from build123d import *

# Parameters (mm, degrees)
EXTRUDE_1_DEPTH          = 4
CUT_EXTRUDE_1_DEPTH      = 3
SKETCH_4_R               = 2.6
CUT_EXTRUDE_9_DEPTH      = 19
CUT_EXTRUDE_9_DEPTH_BACK = 2
SKETCH_5_W               = 0.2
SKETCH_5_H               = 8
CUT_EXTRUDE_11_DEPTH     = 5


with BuildPart() as part:
    # 草圖1 → 填料-伸長1 (new body)
    with BuildSketch(Plane.XY):
        with BuildLine():
            Line((-9, 0), (-9, 43))
            ThreePointArc((-9, 43), (0, 52), (9, 43))
            Line((9, 43), (9, 0))
            Line((9, 0), (-9, 0))
        make_face()
    extrude(amount=EXTRUDE_1_DEPTH)

    # 草圖2 → 除料-伸長1 (cut)
    with BuildSketch(Plane.XY.offset(4)):
        with BuildLine():
            Line((-2.6, 47.145110573), (-5, 33.352358854))
            ThreePointArc((-5, 33.352358854), (-6.5, 29.199046922), (-5, 25.045734991))
            Line((-5, 25.045734991), (-2.656326538, 11.243300615))
            ThreePointArc((-2.656326538, 11.243300615), (0, 9), (2.656326538, 11.243300615))
            Line((2.656326538, 11.243300615), (5, 25.045734991))
            ThreePointArc((5, 25.045734991), (6.5, 29.199046922), (5, 33.352358854))
            Line((5, 33.352358854), (2.6, 47.145110573))
            ThreePointArc((2.6, 47.145110573), (0, 49.331766334), (-2.6, 47.145110573))
        make_face()
    extrude(amount=-CUT_EXTRUDE_1_DEPTH, mode=Mode.SUBTRACT)

    # 草圖4 → 除料-伸長9 (cut, two sides)
    with BuildSketch(Plane.XY) as cut_extrude_9_sk:
        with Locations((0, 29.065156497)):
            Circle(SKETCH_4_R)
    extrude(amount=CUT_EXTRUDE_9_DEPTH, mode=Mode.SUBTRACT)
    extrude(cut_extrude_9_sk.sketch, amount=-CUT_EXTRUDE_9_DEPTH_BACK, mode=Mode.SUBTRACT)

    # 草圖5 → 除料-伸長11 (cut, through all)
    with BuildSketch(Plane.XY):
        with Locations((0, 4)):
            Rectangle(SKETCH_5_W, SKETCH_5_H)
    extrude(amount=CUT_EXTRUDE_11_DEPTH, mode=Mode.SUBTRACT)


solid = part.part
Work out the finished part from the listing and answer in its coordinate system (mm). A direction names the side the tool comes from. Give positions to 0.01 mm unless a question says otherwise; leave off trailing zeros. Loops run counter-clockwise (first coordinate to the right, second up) from the corner with the lowest first, then second, coordinate; pieces in that order, holes last. Notation, with made-up numbers: (34.5, 57) - (56.5, 57) arc R19 ccw to (56.5, 64) - close; hole circle Ø8 at (6, 58.5). An arc over 180 degrees is marked (long way). Answer in a Markdown table with one row per item. Add a question column.
Q1. The part is cut by section A-A (z = 1.8). Determine the outline of the cut face in (x, y), and give its area (3 significant figures).
Q2. This flat-tipped pin is pushed along its axis until it touches: P1, Ø6.5, axis at x = 2.5, y = 28, coming from the +Z side. Where does it stop, or does it pass through?
Q3. The part is cut by section D-D (y = 45). Determine the outline of the cut face in (x, z).
Q4. The part is cut by section C-C (y = 26). Determine the outline of the cut face in (x, z).
Q5. A tool of negligible diameter and unlimited length cuts with its end or side. For faces 1 (the flat face through (0.1, 4, 2)), 2 (the flat face through (9, 22, 2)), 3 (the flat face through (-3.845, 18.241, 2.521)), from which of +Z, -Z, +X, -X, +Y, -Y can it reach the whole face along a straight path? Write none if from no direction.
Q6. Consider line 1 along Y through (x, z) = (0, 0.7); line 2 along X through (y, z) = (7, 2.35); line 3 along X through (y, z) = (21.5, 2.9). Determine where each line is inside the solid, lowest interval first.
Q7. Determine the mould class of faces 4 (the flat face through (6, 26, 4)), 5 (the flat face through (-3.783, 40.345, 2.521)), 6 (the cylindrical face through (6.5, 29.1, 2.5)), 7 (the flat face through (-9, 21, 2)) for opening direction X: released by +X, released by -X, zero draft, split by the parting line, or undercut.
Q8. The part is cut by section B-B (x = 1). Determine the outline of the cut face in (y, z), and give its area (3 significant figures).
Solution:
| question | item | result |
|---|---|---|
| 1 | outline | (-9, 0) - (-0.1, 0) - (-0.1, 8) - (0.1, 8) - (0.1, 0) - (9, 0) - (9, 43) arc R9 ccw to (-9, 43) - close; hole (-5, 25.05) - (-2.66, 11.24) arc R2.69 ccw to (2.66, 11.24) - (5, 25.05) arc R6.5 ccw to (5, 33.35) - (2.6, 47.15) arc R2.64 ccw to (-2.6, 47.15) - (-5, 33.35) arc R6.5 ccw to start |
| 1 | area | 571 mm² |
| 2 | P1 | stops at z = 1 |
| 3 | outline | (-8.77, 0) - (8.77, 0) - (8.77, 4) - (2.97, 4) - (2.97, 1) - (-2.97, 1) - (-2.97, 4) - (-8.77, 4) - close |
| 4 | outline | (-9, 0) - (9, 0) - (9, 4) - (5.66, 4) - (5.66, 1) - (-5.66, 1) - (-5.66, 4) - (-9, 4) - close |
| 5 | face 1 | +Z, -Z, -Y |
| 5 | face 2 | +Z, -Z, +X, +Y, -Y |
| 5 | face 3 | +Z |
| 6 | line 1 | y = 8 to 26.47, 31.67 to 52 |
| 6 | line 2 | x = -9 to -0.1, 0.1 to 9 |
| 6 | line 3 | x = -9 to -4.4, 4.4 to 9 |
| 7 | face 4 | zero draft |
| 7 | face 5 | undercut |
| 7 | face 6 | undercut |
| 7 | face 7 | released by -X |
| 8 | outline | (0, 0) - (26.67, 0) - (26.67, 1) - (9.19, 1) - (9.19, 4) - (0, 4) - close; (31.47, 0) - (51.94, 0) - (51.94, 4) - (49.13, 4) - (49.13, 1) - (31.47, 1) - close |
| 8 | area | 83.1 mm² |
